```python
from build123d import *

# Parameters (mm, degrees)
SKETCH_1_R          = 0.5
SKETCH_1_R_2        = 1.6
SKETCH_1_R_3        = 1.931745927
SKETCH_1_R_4        = 1.598107179
SKETCH_1_R_5        = 1.917728615
EXTRUDE_1_DEPTH     = 1.6
SKETCH_2_R          = 1.6
CUT_EXTRUDE_1_DEPTH = 87.896098877


with BuildPart() as part:
    # 草图1 → 凸台-拉伸1 (new body)
    with BuildSketch(Plane.XY):
        Polygon((0, 0), (66.04, 0), (66.04, -13.34), (68.58, -15.88), (68.58, -48.8), (66.04, -51.34), (66.04, -53.34), (0, -53.34), align=None)
        with Locations((45.731390723, -50.8)):
            Circle(SKETCH_1_R, mode=Mode.SUBTRACT)
        with Locations((63.5, -50.46)):
            Circle(SKETCH_1_R, mode=Mode.SUBTRACT)
        with Locations((43.191390723, -50.8)):
            Circle(SKETCH_1_R, mode=Mode.SUBTRACT)
        with Locations((40.651390723, -50.8)):
            Circle(SKETCH_1_R, mode=Mode.SUBTRACT)
        with Locations((38.111390723, -50.8)):
            Circle(SKETCH_1_R, mode=Mode.SUBTRACT)
        with Locations((35.571390723, -50.8)):
            Circle(SKETCH_1_R, mode=Mode.SUBTRACT)
        with Locations((33.031390723, -50.8)):
            Circle(SKETCH_1_R, mode=Mode.SUBTRACT)
        with Locations((60.96, -50.46)):
            Circle(SKETCH_1_R, mode=Mode.SUBTRACT)
        with Locations((58.42, -50.46)):
            Circle(SKETCH_1_R, mode=Mode.SUBTRACT)
        with Locations((55.88, -50.46)):
            Circle(SKETCH_1_R, mode=Mode.SUBTRACT)
        with Locations((53.34, -50.46)):
            Circle(SKETCH_1_R, mode=Mode.SUBTRACT)
        with Locations((50.8, -50.46)):
            Circle(SKETCH_1_R, mode=Mode.SUBTRACT)
        with Locations((15, -2.54)):
            Circle(SKETCH_1_R_2, mode=Mode.SUBTRACT)
        with Locations((41.656, -2.54)):
            Circle(SKETCH_1_R, mode=Mode.SUBTRACT)
        with Locations((63.5, -2.54)):
            Circle(SKETCH_1_R, mode=Mode.SUBTRACT)
        with Locations((39.116, -2.54)):
            Circle(SKETCH_1_R, mode=Mode.SUBTRACT)
        with Locations((36.576, -2.54)):
            Circle(SKETCH_1_R, mode=Mode.SUBTRACT)
        with Locations((34.036, -2.54)):
            Circle(SKETCH_1_R, mode=Mode.SUBTRACT)
        with Locations((31.496, -2.54)):
            Circle(SKETCH_1_R, mode=Mode.SUBTRACT)
        with Locations((28.956, -2.54)):
            Circle(SKETCH_1_R, mode=Mode.SUBTRACT)
        with Locations((26.416, -2.54)):
            Circle(SKETCH_1_R, mode=Mode.SUBTRACT)
        with Locations((23.876, -2.54)):
            Circle(SKETCH_1_R, mode=Mode.SUBTRACT)
        with Locations((60.96, -2.54)):
            Circle(SKETCH_1_R, mode=Mode.SUBTRACT)
        with Locations((58.42, -2.54)):
            Circle(SKETCH_1_R, mode=Mode.SUBTRACT)
        with Locations((55.88, -2.54)):
            Circle(SKETCH_1_R, mode=Mode.SUBTRACT)
        with Locations((53.34, -2.54)):
            Circle(SKETCH_1_R, mode=Mode.SUBTRACT)
        with Locations((50.8, -2.54)):
            Circle(SKETCH_1_R, mode=Mode.SUBTRACT)
        with Locations((48.26, -2.54)):
            Circle(SKETCH_1_R, mode=Mode.SUBTRACT)
        with Locations((45.72, -2.54)):
            Circle(SKETCH_1_R, mode=Mode.SUBTRACT)
        with Locations((13.97, -50.8)):
            Circle(SKETCH_1_R_3, mode=Mode.SUBTRACT)
        with Locations((65.5, -17.78)):
            Circle(SKETCH_1_R_4, mode=Mode.SUBTRACT)
        with Locations((65.5, -45.72)):
            Circle(SKETCH_1_R_5, mode=Mode.SUBTRACT)
    extrude(amount=EXTRUDE_1_DEPTH)

    # 草图2 → 切除-拉伸1 (cut, through all)
    with BuildSketch(Plane.XY.offset(1.6)):
        with Locations((55.428544368, -16.466121162)):
            Circle(SKETCH_2_R)
        with Locations((35.172593904, -26.466121162)):
            Circle(SKETCH_2_R)
        with Locations((55.428544368, -36.466121162)):
            Circle(SKETCH_2_R)
    extrude(amount=-CUT_EXTRUDE_1_DEPTH, mode=Mode.SUBTRACT)


solid = part.part
```
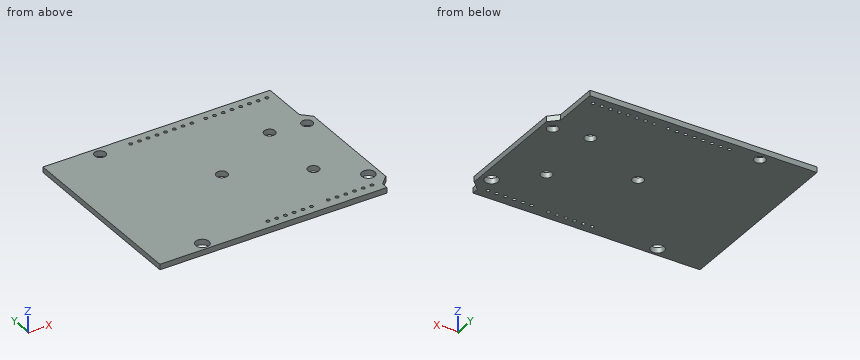
For this review, take the finished solid that the model builds, in its own axes (mm). Coordinates: 2 decimals unless noted, no trailing zeros. Write each loop counter-clockwise with the first axis right and the second up, starting at its lowest first coordinate (ties: lowest second). Pieces come first, ordered by that corner, then holes. Notation, with made-up numbers: (79, -29.75) - (131, -29.75) arc R21 cw to (131, -7.75) - close; hole circle Ø7 at (67, 14.25). An arc over 180 degrees is marked (long way). Put each result on its own line as item: value.
1. Add section B-B, the plane x = 15. Give the boundary of the cut face in (y, z), then the cut area to 3 significant figures.
Values found:
outline: (-53.34, 0) - (-52.43, 0) - (-52.43, 1.6) - (-53.34, 1.6) - close; (-49.17, 0) - (-4.14, 0) - (-4.14, 1.6) - (-49.17, 1.6) - close; (-0.94, 0) - (0, 0) - (0, 1.6) - (-0.94, 1.6) - close
area: 75.0 mm²
2. Add section A-A, the plane y = -45.72. Give the boundary of the cut face in (x, z).
Values found:
outline: (0, 0) - (63.58, 0) - (63.58, 1.6) - (0, 1.6) - close; (67.42, 0) - (68.58, 0) - (68.58, 1.6) - (67.42, 1.6) - close
3. For pin 1 (0.8 mm diameter, centred on y = -52.5, z = 0.5, fed in from +X), flat-tipped, find the tip position at first contact; note if it passes through.
Values found:
pin 1: x = 66.04
4. Add section C-C, the plane z = 0.3. Count the separate pieces of the cut face and the enclosed holes in it, then the cut area to 3 significant figures.
Values found:
separate pieces: 1
enclosed holes: 35
area: 3,530 mm²
5. Add section D-D, the plane y = -12. Give the boundary of the cut face in (x, z), then the cut area to 3 significant figures.
Values found:
outline: (0, 0) - (66.04, 0) - (66.04, 1.6) - (0, 1.6) - close
area: 106 mm²
6. Wall thickness on probe 1 along Y at (x, z) = (58.42, 1.2); probe 2 along Y at (x, z) = (65.5, 0.8); probe 3 along X at (y, z) = (-15.5, 0.2): over which ranges is each line inside the solid? List them lowest first.
Values found:
probe 1: -53.34 to -50.96, -49.96 to -3.04, -2.04 to 0
probe 2: -53.34 to -47.64, -43.8 to -19.38, -16.18 to 0
probe 3: 0 to 54.15, 56.7 to 68.2
